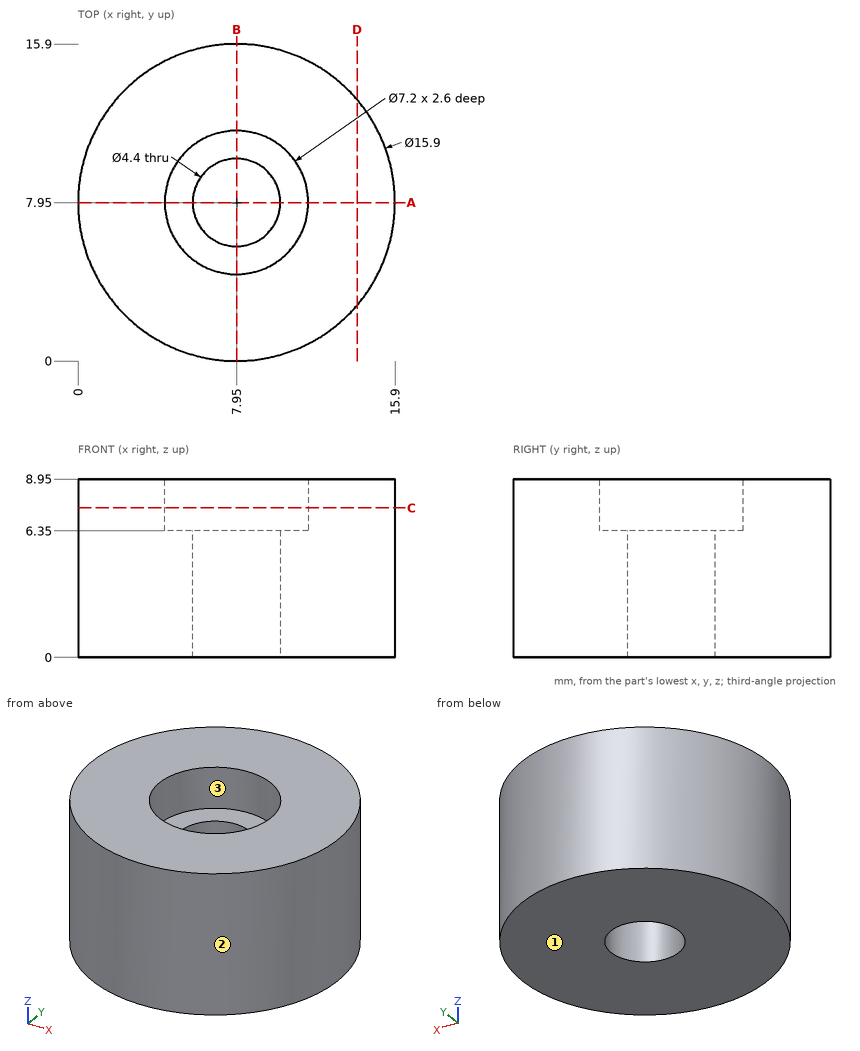
Geometry check sheet. Reference: drawing and pictorial views, mm from the part's lowest x, y, z. Coordinates: 2 decimals unless noted, no trailing zeros. Order: outer loops, then holes, each group sorted by start corner. A loop starts at its lowest first (then second) coordinate and runs counter-clockwise, first axis right, second up. Notation, with made-up numbers: (-39, 15.25) -> (-29, 15.25) arc R13 cw to (-29, 33.25) -> close; hole circle Ø1 at (21.5, 57). An arc over 180 degrees is marked (long way). Write item = value, one per line. Start each with the question number.
1) Cross-section at C-C (z = 7.5). Enter the section's corners in (x, y).
2) Mould release check, pull along Y, two halves, no side actions. Record for the marked faces 1, 2 and 3: +Y half, -Y half, draft (parallel to the pull), parting line (faces both ways), or undercut.
3) Cross-section at A-A (y = 7.95). Enter the section's corners in (x, z), then the cut area to 3 significant figures.
4) Go/stop test with flat-tipped pins: P1, Ø4, axis at y = 12, z = 2.5, coming from the +X side; P2, Ø1.5, axis at x = 9, z = 7.5, coming from the -Y side; P3, Ø3, axis at x = 11, z = 7, coming from the +Y side. Record where each tip stops, or that it passes through.
5) Material ranges on L1, parallel to Y at x = 7.95, z = 7.3; L2, parallel to Y at x = 7.95, z = 2.25; L3, parallel to Z at x = 9, y = 5.25, recorded low to high.
6) Cross-section at D-D (x = 14). Enter the section's corners in (y, z), then the cut area to 3 significant figures.
Ans:
q1.outline = circle Ø15.9 at (7.95, 7.95); hole circle Ø7.2 at (7.95, 7.95)
q2.face_1 = draft
q2.face_2 = parting line
q2.face_3 = undercut
q3.outline = (0, 0) -> (5.75, 0) -> (5.75, 6.35) -> (4.35, 6.35) -> (4.35, 8.95) -> (0, 8.95) -> close; (10.15, 0) -> (15.9, 0) -> (15.9, 8.95) -> (11.55, 8.95) -> (11.55, 6.35) -> (10.15, 6.35) -> close
q3.area = 95.6 mm²
q4.P1 = 15.63
q4.P2 = 0.01
q4.P3 = 15.75
q5.L1 = 0 to 4.35, 11.55 to 15.9
q5.L2 = 0 to 5.75, 10.15 to 15.9
q5.L3 = 0 to 6.35
q6.outline = (2.79, 0) -> (13.11, 0) -> (13.11, 8.95) -> (2.79, 8.95) -> close
q6.area = 92.3 mm²
